from build123d import *

# Parameters (mm, degrees)
F0_R     = 2
F1_DEPTH = 2
F0_W     = 90
F0_H     = 3
F2_DEPTH = 8
F0_R_2   = 1.65
F3_DEPTH = 3
F4_DEPTH = 8


with BuildPart() as f1:
    # F0 (on Top) → F1 (new body)
    with BuildSketch(Plane.XY):
        with BuildLine():
            Line((-25, 10), (-115, 10))
            Line((-115, 10), (-115, -10))
            Line((-115, -10), (115, -10))
            Line((115, -10), (115, 10))
            Line((115, 10), (25.00533, 10))
            Line((25.00533, 10), (19.5469227509, 10))
            ThreePointArc((19.5469227509, 10), (0, -9.5469227509), (-19.5469227509, 10))
            Line((-19.5469227509, 10), (-25, 10))
        make_face()
        with Locations((-106, 2.58)):
            Circle(F0_R, mode=Mode.SUBTRACT)
        with Locations((106, 2.58)):
            Circle(F0_R, mode=Mode.SUBTRACT)
    extrude(amount=F1_DEPTH)

    # F0 (on Top) → F2 (join)
    with BuildSketch(Plane.XY):
        with Locations((-70, 11.5)):
            Rectangle(F0_W, F0_H)
    extrude(amount=F2_DEPTH)

    # F0 (on Top) → F3 (join)
    with BuildSketch(Plane.XY):
        with Locations((-70, 11.5)):
            Rectangle(F0_W, F0_H)
        with BuildLine():
            Line((-25, 10), (-115, 10))
            Line((-115, 10), (-115, -10))
            Line((-115, -10), (115, -10))
            Line((115, -10), (115, 10))
            Line((115, 10), (25.00533, 10))
            Line((25.00533, 10), (19.5469227509, 10))
            ThreePointArc((19.5469227509, 10), (0, -9.5469227509), (-19.5469227509, 10))
            Line((-19.5469227509, 10), (-25, 10))
        make_face()
        with Locations((-106, 2.58)):
            Circle(F0_R, mode=Mode.SUBTRACT)
        with Locations((106, 2.58)):
            Circle(F0_R, mode=Mode.SUBTRACT)
        with BuildLine():
            Line((-25, 13), (-25, 10))
            Line((-25, 10), (-19.5469227509, 10))
            ThreePointArc((-19.5469227509, 10), (-19.4889399629, 11.5044627456), (-19.3153355919, 13))
            Line((-19.3153355919, 13), (-25, 13))
        make_face()
        with BuildLine():
            add(Edge.make_bspline(
                [(-25, 13), (-15.2288932053, 31.7892976505), (-3.8915806674, 54.4419920661), (6.3176813113, 54.2545952389), (17.3850999523, 33.1166154585), (25, 13)],
                knots=[0, 0, 0, 0, 0.4320168298, 0.5736597665, 1, 1, 1, 1], degree=3))
            Line((-25, 13), (-19.3153355919, 13))
            ThreePointArc((-19.3153355919, 13), (0, 29.5469227509), (19.3153355919, 13))
            Line((19.3153355919, 13), (25, 13))
        make_face()
        with Locations((-3.1577504706, 44.9546910822)):
            Circle(F0_R_2, mode=Mode.SUBTRACT)
        with Locations((5.1963478327, 45.1933816075)):
            Circle(F0_R_2, mode=Mode.SUBTRACT)
        with BuildLine():
            ThreePointArc((19.3153355919, 13), (19.4889399629, 11.5044627456), (19.5469227509, 10))
            Line((19.5469227509, 10), (25.00533, 10))
            Line((25.00533, 10), (25, 13))
            Line((25, 13), (19.3153355919, 13))
        make_face()
        Polygon((115, 13), (25, 13), (25.00533, 10), (115, 10), align=None)
    extrude(amount=F3_DEPTH)

    # F0 (on Top) → F4 (join)
    with BuildSketch(Plane.XY):
        Polygon((115, 13), (25, 13), (25.00533, 10), (115, 10), align=None)
    extrude(amount=F4_DEPTH)


solid = f1.part
Model file for the job. Use its own axes, mm. A direction names the side the tool comes from. Give positions to 0.01 mm unless a question says otherwise; leave off trailing zeros. Loops run counter-clockwise (first coordinate to the right, second up) from the corner with the lowest first, then second, coordinate; pieces in that order, holes last.
1) Saw through at C-C (y = 2.58). Write the cut outline in (x, z), plus the area to 3 significant figures.
2) Saw through at A-A (x = 106). Write the cut outline in (y, z).
3) Wall check: line 1 (X direction, y = 10, z = 1.7); line 2 (Z direction, x = -25.5, y = 4); line 3 (Y direction, x = -39.5, z = 1). Give the ranges that are in metal, low to high.
4) Tool access for faces 5 (the flat face through (-71, 13, 4)), 6 (the flat face through (-71, 10, 5)), 7 (the flat face through (71, 13, 4)): list every direction of +Z, -Z, +X, -X, +Y, -Y with a clear straight run to the whole face (end or side of a thin tool).
5) Saw through at D-D (x = -87). Write the cut outline in (y, z).
6) Pull direction X, two halves, no side cores. Call faces 1 (the flat face through (-18, -4, 0)), 2 (the flat face through (115, 4, 2)), 3 (the cylindrical face through (104.5, 3.9, 1.5)), 4 (the cylindrical face through (-107.5, 3.9, 1.5)): +X half, -X half, draft (parallel to the pull), parting line (faces both ways), or undercut.
7) Flat gauge pins, fed straight in: pin 1 Ø3 at (x, y) = (5.2, 45.19) entering from -Z; pin 2 Ø2.5 at (x, z) = (62, 5.5) entering from -Y; pin 3 Ø2.5 at (x, z) = (-72.5, 2.5) entering from +Y; pin 4 Ø6.5 at (x, y) = (106, 2.58) entering from +Z. Where does each tip first touch, or does it go through?
8) Saw through at B-B (z = 6.75). Write the cut outline in (x, y), plus the area to 3 significant figures.
Answer block:
1. outline: (-115, 0) - (-108, 0) - (-108, 3) - (-115, 3) - close; (-104, 0) - (-18.08, 0) - (-18.08, 3) - (-104, 3) - close; (18.08, 0) - (104, 0) - (104, 3) - (18.08, 3) - close; (108, 0) - (115, 0) - (115, 3) - (108, 3) - close
1. area: 557 mm2
2. outline: (-10, 0) - (0.58, 0) - (0.58, 3) - (-10, 3) - close; (4.58, 0) - (13, 0) - (13, 8) - (10, 8) - (10, 3) - (4.58, 3) - close
3. line 1: x = -115 to -19.55, 19.55 to 115
3. line 2: z = 0 to 3
3. line 3: y = -10 to 13
4. face 5: +Z, -Z, -X, +Y
4. face 6: +Z, +X, -X, -Y
4. face 7: +Z, -Z, +X, +Y
5. outline: (-10, 0) - (13, 0) - (13, 8) - (10, 8) - (10, 3) - (-10, 3) - close
6. face 1: draft
6. face 2: +X half
6. face 3: undercut
6. face 4: undercut
7. pin 1: passes through
7. pin 2: stops at y = 10
7. pin 3: stops at y = 13
7. pin 4: stops at z = 3
8. outline: (-115, 10) - (-25, 10) - (-25, 13) - (-115, 13) - close; (25, 13) - (25.01, 10) - (115, 10) - (115, 13) - close
8. area: 540 mm2
